Read the model definition and answer for the solid it produces. Units are mm, in the model's axes. Round coordinates to 2 decimals unless told otherwise and drop trailing zeros. Order: outer loops, then holes, each group sorted by start corner. A loop starts at its lowest first (then second) coordinate and runs counter-clockwise, first axis right, second up. Notation, with made-up numbers: (36.25, -35) -> (79.25, -35) arc R31 ccw to (79.25, -11) -> close; hole circle Ø2 at (-17.5, -4). An arc over 180 degrees is marked (long way). Use a Markdown table: item, result. Add a question column.
1. Consider L1, parallel to Y at x = -205, z = 0.75; L2, parallel to Y at x = 0, z = 0.8; L3, parallel to X at y = 23, z = 2.45. Determine where each line is inside the solid, lowest interval first. Write a range as [from, to].
2. Section A-A, the plane x = 79 is taken. Give the vertices of the cut face in (y, z).
3. Section D-D, the plane x = 0 is taken. Give the vertices of the cut face in (y, z), then the cut area to 3 significant figures.
4. Section C-C, the plane z = 0.45 is taken. Give the number of separate pieces and of enclosed holes in the cut face, then the cut area to 3 significant figures.
5. The mould has two halves that part along X. Classify faces 1 (the face through (-3, 53, 3)), 2 (the face through (2.406, 64.164, 1.479)): +X half, -X half, draft (parallel to the pull), parting line (faces both ways), or undercut.
6. Section B-B, the plane y = -43 is taken. Give the vertices of the cut face in (x, z).
```python
from build123d import *

# Parameters (mm, degrees)
CROQUIS1_W              = 440
CROQUIS1_H              = 230
SALIENTE_EXTRUIR1_DEPTH = 3
CROQUIS2_R              = 3.1
CORTAR_EXTRUIR1_DEPTH   = 4
CROQUIS3_W              = 180
CROQUIS3_H              = 120
CORTAR_EXTRUIR2_DEPTH   = 4
CROQUIS4_R              = 11.1
CORTAR_EXTRUIR3_DEPTH   = 4
CROQUIS5_W              = 13
CROQUIS5_H              = 19
CORTAR_EXTRUIR4_DEPTH   = 4


with BuildPart() as part:
    # Croquis1 → Saliente-Extruir1 (new body)
    with BuildSketch(Plane.XY):
        Rectangle(CROQUIS1_W, CROQUIS1_H)
    extrude(amount=SALIENTE_EXTRUIR1_DEPTH)

    # Croquis2 → Cortar-Extruir1 (cut, through all)
    with BuildSketch(Plane.XY.offset(3)):
        with Locations((-205, 55)):
            Circle(CROQUIS2_R)
        with Locations((-152.5, 100)):
            Circle(CROQUIS2_R)
        with Locations((152.5, 100)):
            Circle(CROQUIS2_R)
        with Locations((-205, -55)):
            Circle(CROQUIS2_R)
        with Locations((205, -55)):
            Circle(CROQUIS2_R)
        with Locations((205, 55)):
            Circle(CROQUIS2_R)
        with Locations((152.5, -100)):
            Circle(CROQUIS2_R)
        with Locations((-152.5, -100)):
            Circle(CROQUIS2_R)
    extrude(amount=-CORTAR_EXTRUIR1_DEPTH, mode=Mode.SUBTRACT)

    # Croquis3 → Cortar-Extruir2 (cut, through all)
    with BuildSketch(Plane(origin=(0, 0, 0), x_dir=(-1, 0, 0), z_dir=(0, 0, -1))):
        with Locations((0, -20)):
            Rectangle(CROQUIS3_W, CROQUIS3_H)
    extrude(amount=-CORTAR_EXTRUIR2_DEPTH, mode=Mode.SUBTRACT)

    # Croquis4 → Cortar-Extruir3 (cut, through all)
    with BuildSketch(Plane(origin=(0, 0, 0), x_dir=(-1, 0, 0), z_dir=(0, 0, -1))):
        with Locations((0, 75)):
            Circle(CROQUIS4_R)
    extrude(amount=-CORTAR_EXTRUIR3_DEPTH, mode=Mode.SUBTRACT)

    # Croquis5 → Cortar-Extruir4 (cut, through all)
    with BuildSketch(Plane(origin=(0, 0, 0), x_dir=(-1, 0, 0), z_dir=(0, 0, -1))):
        with Locations((-110, -40.5)):
            Rectangle(CROQUIS5_W, CROQUIS5_H)
    extrude(amount=-CORTAR_EXTRUIR4_DEPTH, mode=Mode.SUBTRACT)


solid = part.part
```
Verdict:
| question | item | result |
|---|---|---|
| 1 | L1 | y = [-115, -58.1], [-51.9, 51.9], [58.1, 115] |
| 1 | L2 | y = [-115, -80], [40, 63.9], [86.1, 115] |
| 1 | L3 | x = [-220, -90], [90, 220] |
| 2 | outline | (-115, 0) -> (-80, 0) -> (-80, 3) -> (-115, 3) -> close; (40, 0) -> (115, 0) -> (115, 3) -> (40, 3) -> close |
| 3 | outline | (-115, 0) -> (-80, 0) -> (-80, 3) -> (-115, 3) -> close; (40, 0) -> (63.9, 0) -> (63.9, 3) -> (40, 3) -> close; (86.1, 0) -> (115, 0) -> (115, 3) -> (86.1, 3) -> close |
| 3 | area | 263 mm2 |
| 4 | separate pieces | 1 |
| 4 | enclosed holes | 11 |
| 4 | area | 78,700 mm2 |
| 5 | face 1 | draft |
| 5 | face 2 | undercut |
| 6 | outline | (-220, 0) -> (-90, 0) -> (-90, 3) -> (-220, 3) -> close; (90, 0) -> (103.5, 0) -> (103.5, 3) -> (90, 3) -> close; (116.5, 0) -> (220, 0) -> (220, 3) -> (116.5, 3) -> close |
